The listing builds one solid part. Answer for the finished solid, in the listing's coordinates (mm). A direction names the side the tool comes from. Round coordinates to 2 decimals unless told otherwise and drop trailing zeros. Write each loop counter-clockwise with the first axis right and the second up, starting at its lowest first coordinate (ties: lowest second). Pieces come first, ordered by that corner, then holes.
Item 1: Each of these flat-tipped pins is pushed along its axis until it touches: pin 1 (1 mm diameter, centred on y = 1.5, z = -36.5, fed in from +X); pin 2 (1 mm diameter, centred on x = 81, y = 5, fed in from +Z). Where does it stop, or does it pass through?
Item 2: Find section C-C on y = 3.95. Give the number of separate pieces and of enclosed holes in the cut face, then the cut area to 3 significant figures.
Item 3: Find section A-A on z = -5.5. Give the vertices of the cut face in (x, y).
Item 4: Find the intervals of material crossed by probe 1 along Z at (x, y) = (80, 4.4); probe 2 along X at (y, z) = (1.85, 61.5); probe 3 along X at (y, z) = (3.65, 58.5), in increasing order.
Item 5: A tool of negligible diameter and unlimited length cuts with its end or side. For faces 1 (the face through (168.6, 3, 0)), 2 (the face through (147.339, 2.958, -27.792)), from which of +Z, -Z, +X, -X, +Y, -Y can it reach the whole face along a straight path? Write none if from no direction.
Item 6: Find section D-D on x = 133.5. Give the vertices of the cut face in (y, z), then the cut area to 3 significant figures.
Item 7: For a pull along Z with two mould halves and no side action, classify faces 3 (the face through (120.474, 2.958, -35.902)), 4 (the face through (-121.4, 3, 0)), 5 (the face through (147.939, 2.958, 27.634)) as +Z half, -Z half, draft (parallel to the pull), parting line (faces both ways), or undercut.
Item 8: Find section B-B on x = -48. Give the vertices of the cut face in (y, z), then the cut area to 3 significant figures.
```python
from build123d import *

# Parameters (mm, degrees)
BOSS_EXTRUDE2_DEPTH = 6
SKETCH2_R           = 5
CUT_EXTRUDE2_DEPTH  = 6


with BuildPart() as part:
    # Sketch1 → Boss-Extrude2 (new body)
    with BuildSketch(Plane(origin=(0, 0, 0), x_dir=(1, 0, 0), z_dir=(0, 1, 0))):
        with BuildLine():
            Line((-91, -69.5), (-126, -22.833333333))
            ThreePointArc((-126, -22.833333333), (-128.973665961, -17.157888654), (-130, -10.833333333))
            Line((-130, -10.833333333), (-130, 10.833333333))
            ThreePointArc((-130, 10.833333333), (-128.973665961, 17.157888654), (-126, 22.833333333))
            Line((-126, 22.833333333), (-91, 69.5))
            ThreePointArc((-91, 69.5), (-83.94427191, 75.38854382), (-75, 77.5))
            Line((-75, 77.5), (75.561511123, 77.5))
            ThreePointArc((75.561511123, 77.5), (84.097233086, 75.587052014), (91.000115835, 70.214145057))
            Line((91.000115835, 70.214145057), (115.898546704, 39.980336145))
            ThreePointArc((115.898546704, 39.980336145), (120.54751552, 35.854535916), (126.238632031, 33.355269737))
            Line((126.238632031, 33.355269737), (169.039407754, 22.071428865))
            ThreePointArc((169.039407754, 22.071428865), (173.337004893, 19.218609112), (175, 14.335744279))
            Line((175, 14.335744279), (175, -14.335744279))
            ThreePointArc((175, -14.335744279), (173.337004893, -19.218609112), (169.039407754, -22.071428865))
            Line((169.039407754, -22.071428865), (126.238632031, -33.355269737))
            ThreePointArc((126.238632031, -33.355269737), (120.54751552, -35.854535916), (115.898546704, -39.980336145))
            Line((115.898546704, -39.980336145), (91.000115835, -70.214145057))
            ThreePointArc((91.000115835, -70.214145057), (84.097233086, -75.587052014), (75.561511123, -77.5))
            Line((75.561511123, -77.5), (-75, -77.5))
            ThreePointArc((-75, -77.5), (-83.94427191, -75.38854382), (-91, -69.5))
        make_face()
    extrude(amount=BOSS_EXTRUDE2_DEPTH)

    # Sketch2 → Cut-Extrude2 (cut)
    with BuildSketch(Plane(origin=(0, 6, 0), x_dir=(1, 0, 0), z_dir=(0, 1, 0))):
        with Locations((80, -61.5)):
            Circle(SKETCH2_R)
        with BuildLine():
            Line((168.6, 15), (168.6, -15))
            ThreePointArc((168.6, -15), (166.5, -17.1), (164.4, -15))
            Line((164.4, -15), (164.4, 15))
            ThreePointArc((164.4, 15), (166.5, 17.1), (168.6, 15))
        make_face()
        with BuildLine():
            Line((-121.4, 15), (-121.4, -15))
            ThreePointArc((-121.4, -15), (-123.5, -17.1), (-125.6, -15))
            Line((-125.6, -15), (-125.6, 15))
            ThreePointArc((-125.6, 15), (-123.5, 17.1), (-121.4, 15))
        make_face()
        with BuildLine():
            Line((-92.5, 47), (92.5, 47))
            ThreePointArc((92.5, 47), (94.5, 45), (92.5, 43))
            Line((92.5, 43), (-92.5, 43))
            ThreePointArc((-92.5, 43), (-94.5, 45), (-92.5, 47))
        make_face()
        with BuildLine():
            Line((-92.5, -43), (92.5, -43))
            ThreePointArc((92.5, -43), (94.5, -45), (92.5, -47))
            Line((92.5, -47), (-92.5, -47))
            ThreePointArc((-92.5, -47), (-94.5, -45), (-92.5, -43))
        make_face()
        with BuildLine():
            Line((-92.5, 27), (92.5, 27))
            ThreePointArc((92.5, 27), (94.5, 25), (92.5, 23))
            Line((92.5, 23), (-92.5, 23))
            ThreePointArc((-92.5, 23), (-94.5, 25), (-92.5, 27))
        make_face()
        with BuildLine():
            Line((-92.5, -23), (92.5, -23))
            ThreePointArc((92.5, -23), (94.5, -25), (92.5, -27))
            Line((92.5, -27), (-92.5, -27))
            ThreePointArc((-92.5, -27), (-94.5, -25), (-92.5, -23))
        make_face()
        with BuildLine():
            Line((-75, 70), (75, 70))
            ThreePointArc((75, 70), (77, 68), (75, 66))
            Line((75, 66), (-75, 66))
            ThreePointArc((-75, 66), (-77, 68), (-75, 70))
        make_face()
        with BuildLine():
            Line((-77.53734134, -59.5), (67.46265866, -59.5))
            ThreePointArc((67.46265866, -59.5), (69.46265866, -61.5), (67.46265866, -63.5))
            Line((67.46265866, -63.5), (-77.53734134, -63.5))
            ThreePointArc((-77.53734134, -63.5), (-79.53734134, -61.5), (-77.53734134, -59.5))
        make_face()
    extrude(amount=-CUT_EXTRUDE2_DEPTH, mode=Mode.SUBTRACT)


solid = part.part
```
Check values:
1. pin 1: stops at x = 120.32
1. pin 2: stops at z = 76.88
2. separate pieces: 1
2. enclosed holes: 9
2. area: 33,000 mm2
3. outline: (-130, 0) - (-125.6, 0) - (-125.6, 6) - (-130, 6) - close; (-121.4, 0) - (164.4, 0) - (164.4, 6) - (-121.4, 6) - close; (168.6, 0) - (175, 0) - (175, 6) - (168.6, 6) - close
4. probe 1: z = -77 to -47, -43 to -27, -23 to 23, 27 to 43, 47 to 56.5, 66.5 to 77
4. probe 2: x = -97 to -79.54, 69.46 to 75, 85 to 98.18
4. probe 3: x = -99.25 to 76, 84 to 100.65
5. face 1: +Y, -Y
5. face 2: -Z, +X, +Y, -Y
6. outline: (0, -31.44) - (6, -31.44) - (6, 31.44) - (0, 31.44) - close
6. area: 377 mm2
7. face 3: -Z half
7. face 4: undercut
7. face 5: +Z half
8. outline: (0, -77.5) - (6, -77.5) - (6, -70) - (0, -70) - close; (0, -66) - (6, -66) - (6, -47) - (0, -47) - close; (0, -43) - (6, -43) - (6, -27) - (0, -27) - close; (0, -23) - (6, -23) - (6, 23) - (0, 23) - close; (0, 27) - (6, 27) - (6, 43) - (0, 43) - close; (0, 47) - (6, 47) - (6, 59.5) - (0, 59.5) - close; (0, 63.5) - (6, 63.5) - (6, 77.5) - (0, 77.5) - close
8. area: 786 mm2
